Design review of the part built by this model. Coordinates are the model's own, in mm. Face numbers are marked on the shaded views. A direction names the side the tool comes from. Give positions to 0.01 mm unless a question says otherwise; leave off trailing zeros. Write each loop counter-clockwise with the first axis right and the second up, starting at its lowest first coordinate (ties: lowest second). Pieces come first, ordered by that corner, then holes. Notation, with made-up numbers: M 1,-33 L 41,-33 A30 cw 41,3 Z; hole C 47.25,79 d9. An arc over 180 degrees is marked long. Use one line per item in the form item = value. Start each with the question number.
from build123d import *

# Parameters (mm, degrees)
CUT_EXTRUDE1_DEPTH      = 118.447860772
CUT_EXTRUDE1_DEPTH_BACK = 118.447860772
SKETCH2_R               = 19
CUT_EXTRUDE3_START      = -31
CUT_EXTRUDE3_DEPTH      = 172.206989852
CIRPATTERN1_COUNT       = 4


with BuildPart() as part:
    # Sketch1 → Revolve1 (revolve)
    with BuildSketch(Plane.XY):
        with BuildLine():
            Line((-25, 0), (112, 0))
            Line((112, 0), (112, 12.5))
            Line((112, 12.5), (21.650635095, 12.5))
            ThreePointArc((21.650635095, 12.5), (-6.470476128, 24.148145657), (-25, 0))
        make_face()
    revolve(axis=Axis((-25, 0, 0), (1, 0, 0)))

    # Sketch2 → Cut-Extrude1 (cut, two sides: drawn at the far end of the back side and taken through both)
    with BuildSketch(Plane.XY.offset(-CUT_EXTRUDE1_DEPTH_BACK)):
        Circle(SKETCH2_R)
    extrude(amount=CUT_EXTRUDE1_DEPTH + CUT_EXTRUDE1_DEPTH_BACK, mode=Mode.SUBTRACT)

    # Sketch4 → Cut-Extrude3 (cut)
    with BuildSketch(Plane(origin=(112, 0, 0), x_dir=(0, 0, -1), z_dir=(1, 0, 0)).offset(CUT_EXTRUDE3_START)):
        with BuildLine():
            Line((-7, 10.356157589), (7, 10.356157589))
            ThreePointArc((7, 10.356157589), (0, 12.5), (-7, 10.356157589))
        make_face()
    cut_extrude3 = extrude(amount=CUT_EXTRUDE3_DEPTH, mode=Mode.SUBTRACT)

    # CirPattern1: Cut-Extrude3 ×4 about axis
    cirpattern1_axis = Axis((0, 0, 0), (1, 0, 0))
    for i in range(1, CIRPATTERN1_COUNT):
        add(cut_extrude3.rotate(cirpattern1_axis, i * 360 / CIRPATTERN1_COUNT), mode=Mode.SUBTRACT)


solid = part.part
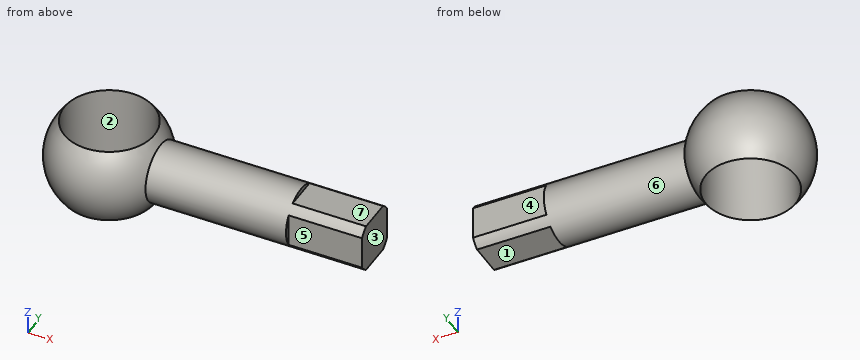
1. Clearance check with flat-ended pins moving along their axes: pin 1 Ø6 at (y, z) = (-17, 7) entering from -X; pin 2 Ø3 at (x, y) = (36, 12.5) entering from +Z; pin 3 Ø5 at (x, z) = (27.5, 5.5) entering from -Y. State where each tip first meets the part, or that it passes through.
2. For the marked faces 4, 5, 6 and 7, list the 3-axis set-ups (+Z, -Z, +X, -X, +Y, -Y) from which the entire face can be reached by the end or side of a thin tool; tool diameter is ignored.
3. We need section D-D (x = 0). State the section outline as (y, z) points, and give its area (3 significant figures).
4. We need section B-B (z = 0). State the section outline as (x, y) points, and give its area (3 significant figures).
5. We need section A-A (y = 0). State the section outline as (x, z) points, and give its area (3 significant figures).
6. Draft analysis for pull direction X (two halves, no side actions). For the marked faces 1, 2 and 3, state which applies: pulls with the +X half, pulls with the -X half, needs draft (parallel to the pull), parting line crosses it, or undercut.
7. We need section C-C (x = 98.5). State the section outline as (y, z) points.
8. To check wall thickness, follow L1, parallel to X at y = 14.5, z = 10; L2, parallel to X at y = 0, z = 10; L3, parallel to Y at x = 80, z = 0.5. State the ranges of each line that lie inside material, in increasing order.
Answer block:
q1.pin_1 = -19.71
q1.pin_2 = 5.94
q1.pin_3 = -12.13
q2.face_4 = +Z, -Z, +X, +Y
q2.face_5 = +Z, -Z, +X, -Y
q2.face_6 = +X
q2.face_7 = +Z, +X, +Y, -Y
q3.outline = M -19,-16.25 L -19,16.25 A25 ccw Z; M 19,-16.25 A25 ccw 19,16.25 Z
q3.area = 267 mm^2
q4.outline = M 21.65,-12.5 L 81,-12.5 L 81,-10.36 L 112,-10.36 L 112,10.36 L 81,10.36 L 81,12.5 L 21.65,12.5 A25 ccw long Z; hole C 0,0 d38
q4.area = 2,900 mm^2
q5.outline = M -19,-16.25 L -19,16.25 A25 ccw Z; M 19,-16.25 A25 ccw 21.65,-12.5 L 81,-12.5 L 81,-10.36 L 112,-10.36 L 112,10.36 L 81,10.36 L 81,12.5 L 21.65,12.5 A25 ccw 19,16.25 Z
q5.area = 2,340 mm^2
q6.face_1 = needs draft
q6.face_2 = undercut
q6.face_3 = pulls with the +X half
q7.outline = M -10.36,-7 A12.5 ccw -7,-10.36 L 7,-10.36 A12.5 ccw 10.36,-7 L 10.36,7 A12.5 ccw 7,10.36 L -7,10.36 A12.5 ccw -10.36,7 Z
q8.L1 = -17.74 to -12.28, 12.28 to 17.74
q8.L2 = -22.91 to -19, 19 to 112
q8.L3 = -12.49 to 12.49
